Input: dimensioned drawing with shaded views. Units: mm. Origin: part minimum x, y, z. Give positions to 0.01 mm unless a question says otherwise; leave off trailing zeros. Order: outer loops, then holes, each group sorted by start corner. A loop starts at its lowest first (then second) coordinate and runs counter-clockwise, first axis right, second up. Notation, with made-up numbers: M 0,-29 L 48,-29 A17 ccw 48,-7 Z; hole C 66,-35.75 d8. An arc over 180 degrees is marked long. Answer in a Markdown table with one row per item. Add a question column.
(1) Pin query (flat end, axial travel): P1, Ø8, axis at x = 6.5, z = 43, coming from the +Y side; P2, Ø4, axis at x = 19.5, z = 25, coming from the +Y side. Return the tip coordinate at first contact, or that it passes through.
(2) Mould query, pull axis X, two halves, no side actions, for the marked faces 1 and 2. Classes: pulls with the +X half, pulls with the -X half, needs draft (parallel to the pull), parting line crosses it, or undercut.
(3) Material intervals for line 1 along Z through (x, y) = (29, 1.95); line 2 along Y through (x, z) = (16, 43.5); line 3 along X through (y, z) = (3.5, 25), sorted ascending.
(4) Section query C-C, the plane x = 19.5. Return loops of the section in (y, z) (1 decimal).
(5) Section query A-A, the plane z = 4. Return loops of the section in (x, y).
(6) Section query D-D, the plane x = 4. Return loops of the section in (y, z), plus the area to 3 significant figures.
(7) Section query B-B, the plane y = 1.4. Count the separate pieces of the cut face and the enclosed holes in it, plus the area to 3 significant figures.
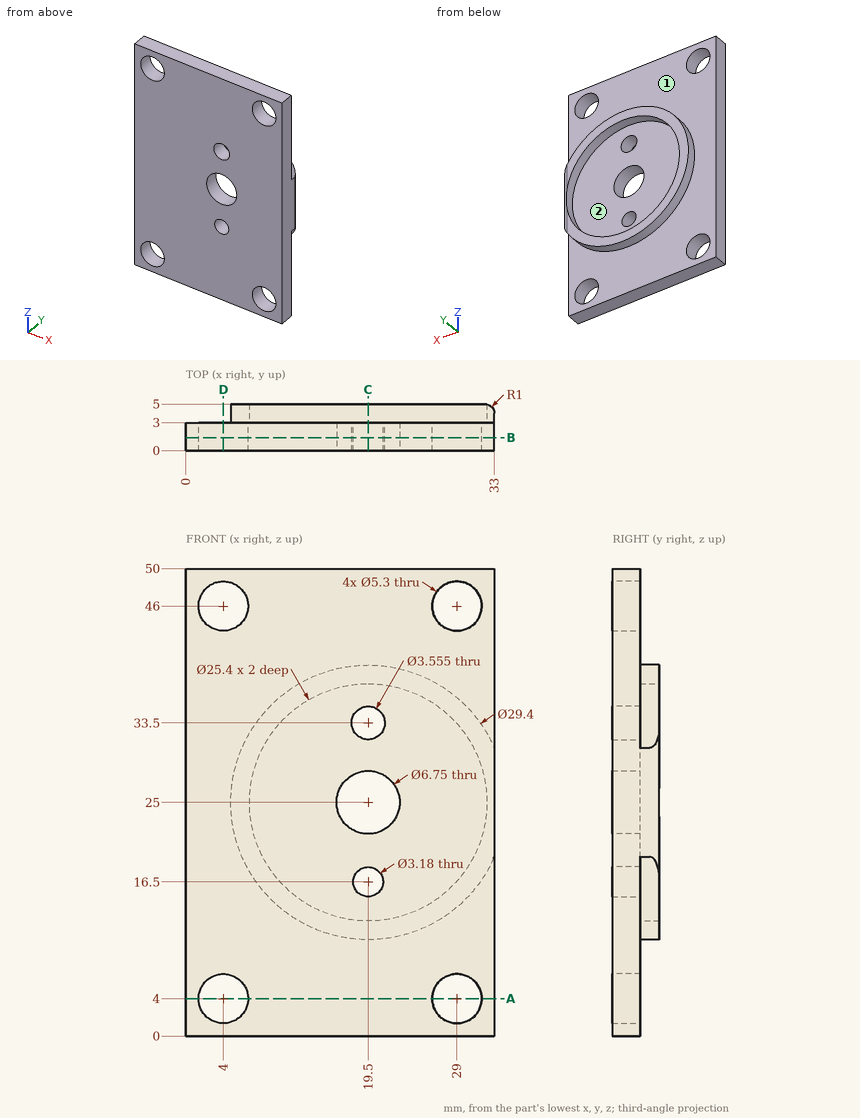
Values follow:
| question | item | result |
|---|---|---|
| 1 | P1 | stops at y = 3 |
| 1 | P2 | passes through |
| 2 | face 1 | needs draft |
| 2 | face 2 | undercut |
| 3 | line 1 | z = 0 to 1.35, 6.65 to 43.35, 48.65 to 50 |
| 3 | line 2 | y = 0 to 3 |
| 3 | line 3 | x = 4.8 to 6.8, 32.2 to 33 |
| 4 | outline | M 0,0 L 3,0 L 3,10.3 L 5,10.3 L 5,12.3 L 3,12.3 L 3,14.9 L 0,14.9 Z; M 0,18.1 L 3,18.1 L 3,21.6 L 0,21.6 Z; M 0,28.4 L 3,28.4 L 3,31.7 L 0,31.7 Z; M 0,35.3 L 3,35.3 L 3,37.7 L 5,37.7 L 5,39.7 L 3,39.7 L 3,50 L 0,50 Z |
| 5 | outline | M 0,0 L 1.35,0 L 1.35,3 L 0,3 Z; M 6.65,0 L 26.35,0 L 26.35,3 L 6.65,3 Z; M 31.65,0 L 33,0 L 33,3 L 31.65,3 Z |
| 6 | outline | M 0,0 L 3,0 L 3,1.35 L 0,1.35 Z; M 0,6.65 L 3,6.65 L 3,43.35 L 0,43.35 Z; M 0,48.65 L 3,48.65 L 3,50 L 0,50 Z |
| 6 | area | 118 mm² |
| 7 | separate pieces | 1 |
| 7 | enclosed holes | 7 |
| 7 | area | 1,510 mm² |
